```python
from build123d import *

# Parameters (mm, degrees)
F0_W           = 97
F0_H           = 125
F0_R           = 7.367785
F1_DEPTH       = 1.5
F3_D           = 2
F3_CSINK_D     = 4
F3_CSINK_ANGLE = 90


# Not quite as in the source:
# - a feature names something its author has since deleted; it is built from what else it names


with BuildPart() as f1:
    # F0 (on Front) → F1 (new body)
    with BuildSketch(Plane.XZ):
        Rectangle(F0_W, F0_H)
        with BuildLine():
            Line((-34.0249225795, -7.10684), (-10.5249225795, -7.10684))
            ThreePointArc((-10.5249225795, -7.10684), (-5.5751751112, -9.1570925317), (-3.5249225795, -14.10684))
            Line((-3.5249225795, -14.10684), (-3.5249225795, -45.5))
            ThreePointArc((-3.5249225795, -45.5), (-5.5751751112, -50.4497474683), (-10.5249225795, -52.5))
            Line((-10.5249225795, -52.5), (-34.0249225795, -52.5))
            ThreePointArc((-34.0249225795, -52.5), (-38.9746700478, -50.4497474683), (-41.0249225795, -45.5))
            Line((-41.0249225795, -45.5), (-41.0249225795, -14.10684))
            ThreePointArc((-41.0249225795, -14.10684), (-38.9746700478, -9.1570925317), (-34.0249225795, -7.10684))
        make_face(mode=Mode.SUBTRACT)
        with BuildLine():
            ThreePointArc((41.0249225795, -45.5), (38.9746700478, -50.4497474683), (34.0249225795, -52.5))
            Line((34.0249225795, -52.5), (10.5249225795, -52.5))
            ThreePointArc((10.5249225795, -52.5), (5.5751751112, -50.4497474683), (3.5249225795, -45.5))
            Line((3.5249225795, -45.5), (3.5249225795, -14.10684))
            ThreePointArc((3.5249225795, -14.10684), (5.5751751112, -9.1570925317), (10.5249225795, -7.10684))
            Line((10.5249225795, -7.10684), (34.0249225795, -7.10684))
            ThreePointArc((34.0249225795, -7.10684), (38.9746700478, -9.1570925317), (41.0249225795, -14.10684))
            Line((41.0249225795, -14.10684), (41.0249225795, -45.5))
        make_face(mode=Mode.SUBTRACT)
        with BuildLine():
            ThreePointArc((-3.5249225795, 14.10684), (-5.5751751112, 9.1570925317), (-10.5249225795, 7.10684))
            Line((-10.5249225795, 7.10684), (-34.0249225795, 7.10684))
            ThreePointArc((-34.0249225795, 7.10684), (-38.9746700478, 9.1570925317), (-41.0249225795, 14.10684))
            Line((-41.0249225795, 14.10684), (-41.0249225795, 45.5))
            ThreePointArc((-41.0249225795, 45.5), (-38.9746700478, 50.4497474683), (-34.0249225795, 52.5))
            Line((-34.0249225795, 52.5), (-10.5249225795, 52.5))
            ThreePointArc((-10.5249225795, 52.5), (-5.5751751112, 50.4497474683), (-3.5249225795, 45.5))
            Line((-3.5249225795, 45.5), (-3.5249225795, 14.10684))
        make_face(mode=Mode.SUBTRACT)
        Circle(F0_R, mode=Mode.SUBTRACT)
        with BuildLine():
            ThreePointArc((10.5249225795, 7.10684), (5.5751751112, 9.1570925317), (3.5249225795, 14.10684))
            Line((3.5249225795, 14.10684), (3.5249225795, 45.5))
            ThreePointArc((3.5249225795, 45.5), (5.5751751112, 50.4497474683), (10.5249225795, 52.5))
            Line((10.5249225795, 52.5), (34.0249225795, 52.5))
            ThreePointArc((34.0249225795, 52.5), (38.9746700478, 50.4497474683), (41.0249225795, 45.5))
            Line((41.0249225795, 45.5), (41.0249225795, 14.10684))
            ThreePointArc((41.0249225795, 14.10684), (38.9746700478, 9.1570925317), (34.0249225795, 7.10684))
            Line((34.0249225795, 7.10684), (10.5249225795, 7.10684))
        make_face(mode=Mode.SUBTRACT)
    extrude(amount=F1_DEPTH)

    # F3 (through all)
    with Locations(Plane.XZ.offset(1.5)):
        with Locations((-43.5, -59.5), (43.5, -59.5), (43.5, 59.5), (-43.5, 59.5)):
            CounterSinkHole(F3_D / 2, F3_CSINK_D / 2, counter_sink_angle=F3_CSINK_ANGLE)


solid = f1.part
```
For this review, take the finished solid that the model builds, in its own axes (mm). A direction names the side the tool comes from. Round coordinates to 2 decimals unless told otherwise and drop trailing zeros. Write each loop counter-clockwise with the first axis right and the second up, starting at its lowest first coordinate (ties: lowest second). Pieces come first, ordered by that corner, then holes. Notation, with made-up numbers: (-16, -17) - (34, -17) arc R27 cw to (34, 2) - close; hole circle Ø8 at (38, 8). An arc over 180 degrees is marked (long way). Put each result on its own line as item: value.
Q1. Machinability: for faces 3 (the face through (-5.63, -0.74, 50.504)), 4 (the face through (10, 0, 1)), which of the approach directions +Z, -Z, +X, -X, +Y, -Y give a long, thin tool a straight path to every point of the face, cutting with its end or side? Answer none if there is none.
Solved:
face 3: +Y, -Y
face 4: +Z, -Z, +X, -X, +Y
Q2. We need section D-D (y = -0.9). Count the separate pieces of the cut face and the enclosed holes in it, and give its area (3 significant figures).
Solved:
separate pieces: 1
enclosed holes: 9
area: 5,290 mm2
Q3. We need section A-A (x = 24). Give the boundary of the cut face in (y, z), and give its area (3 significant figures).
Solved:
outline: (-1.5, -62.5) - (0, -62.5) - (0, -52.5) - (-1.5, -52.5) - close; (-1.5, -7.11) - (0, -7.11) - (0, 7.11) - (-1.5, 7.11) - close; (-1.5, 52.5) - (0, 52.5) - (0, 62.5) - (-1.5, 62.5) - close
area: 51.3 mm2
Q4. Insertion check: pin 1 Ø1.8 at (x, z) = (43.5, 59.5) entering from -Y; pin 2 Ø2.5 at (x, z) = (-43.5, 59.5) entering from -Y. Each pin has a flat end and moves straight along its axis. Give the tip position at first contact, or say it passes through.
Solved:
pin 1: passes through
pin 2: stops at y = -0.75
Q5. We need section B-B (z = 0). Give the boundary of the cut face in (x, y), and give its area (3 significant figures).
Solved:
outline: (-48.5, -1.5) - (-7.37, -1.5) - (-7.37, 0) - (-48.5, 0) - close; (7.37, -1.5) - (48.5, -1.5) - (48.5, 0) - (7.37, 0) - close
area: 123 mm2
Q6. Wall thickness on probe 1 along X at (y, z) = (-0.3, -45.5); probe 2 along X at (y, z) = (-0.4, 59.5); probe 3 along Z at (x, y) = (-21.5, -1.3): over which ranges is each line inside the solid? List them lowest first.
Solved:
probe 1: x = -48.5 to -41.02, -3.52 to 3.52, 41.02 to 48.5
probe 2: x = -48.5 to -44.5, -42.5 to 42.5, 44.5 to 48.5
probe 3: z = -62.5 to -52.5, -7.11 to 7.11, 52.5 to 62.5
Q7. Mouldability with a two-part tool opening along Z and no side actions: class faces 1 (the face through (-5.521, -0.74, 9.212)), 2 (the face through (10, -1.5, 1)) as released by +Z, released by -Z, zero draft, split by the parting line, or undercut.
Solved:
face 1: undercut
face 2: zero draft
Q8. We need section C-C (z = 24). Give the boundary of the cut face in (x, y), and give its area (3 significant figures).
Solved:
outline: (-48.5, -1.5) - (-41.02, -1.5) - (-41.02, 0) - (-48.5, 0) - close; (-3.52, -1.5) - (3.52, -1.5) - (3.52, 0) - (-3.52, 0) - close; (41.02, -1.5) - (48.5, -1.5) - (48.5, 0) - (41.02, 0) - close
area: 33.0 mm2
